```python
from build123d import *

# Parameters (mm, degrees)
SKETCH_1_W          = 320
SKETCH_1_H          = 121
EXTRUDE_1_DEPTH     = 4
SKETCH_2_W          = 5
SKETCH_2_H          = 30
CUT_EXTRUDE_1_DEPTH = 343.135937896
SKETCH_3_R          = 1.5
CUT_EXTRUDE_2_DEPTH = 343.135937896
SKETCH_4_R          = 1.5
CUT_EXTRUDE_3_DEPTH = 343.135937896
SKETCH_6_R          = 2
CUT_EXTRUDE_5_DEPTH = 343.135937896
SKETCH_5_W          = 250
SKETCH_5_H          = 30
CUT_EXTRUDE_4_DEPTH = 343.135937896


with BuildPart() as part:
    # 草图1 → 凸台-拉伸1 (new body)
    with BuildSketch(Plane.XY):
        with Locations((160, 60.5)):
            Rectangle(SKETCH_1_W, SKETCH_1_H)
    extrude(amount=EXTRUDE_1_DEPTH)

    # 草图2 → 切除-拉伸1 (cut, through all)
    with BuildSketch(Plane.XY.offset(4)):
        with Locations((32.5, 15)):
            Rectangle(SKETCH_2_W, SKETCH_2_H)
        with Locations((287.5, 15)):
            Rectangle(SKETCH_2_W, SKETCH_2_H)
    extrude(amount=-CUT_EXTRUDE_1_DEPTH, mode=Mode.SUBTRACT)

    # 草图3 → 切除-拉伸2 (cut, through all)
    with BuildSketch(Plane.XY.offset(4)):
        with Locations((40, 116)):
            Circle(SKETCH_3_R)
        with Locations((60, 116)):
            Circle(SKETCH_3_R)
        with Locations((140, 116)):
            Circle(SKETCH_3_R)
        with Locations((160, 116)):
            Circle(SKETCH_3_R)
        with Locations(Location((260, 116, 0), (0, 0, 180))):
            Circle(SKETCH_3_R)
        with Locations(Location((280, 116, 0), (0, 0, 180))):
            Circle(SKETCH_3_R)
        with Locations(Location((180, 116, 0), (0, 0, 180))):
            Circle(SKETCH_3_R)
    extrude(amount=-CUT_EXTRUDE_2_DEPTH, mode=Mode.SUBTRACT)

    # 草图4 → 切除-拉伸3 (cut, through all)
    with BuildSketch(Plane.XY.offset(4)):
        with Locations((5, 90)):
            Circle(SKETCH_4_R)
        with Locations((25, 90)):
            Circle(SKETCH_4_R)
        with Locations((5, 10)):
            Circle(SKETCH_4_R)
        with Locations((25, 10)):
            Circle(SKETCH_4_R)
        with Locations(Location((295, 10, 0), (0, 0, 180))):
            Circle(SKETCH_4_R)
        with Locations(Location((315, 10, 0), (0, 0, 180))):
            Circle(SKETCH_4_R)
        with Locations(Location((295, 90, 0), (0, 0, 180))):
            Circle(SKETCH_4_R)
        with Locations(Location((315, 90, 0), (0, 0, 180))):
            Circle(SKETCH_4_R)
    extrude(amount=-CUT_EXTRUDE_3_DEPTH, mode=Mode.SUBTRACT)

    # 草图6 → 切除-拉伸5 (cut, through all)
    with BuildSketch(Plane.XY.offset(4)):
        with Locations((112.5, 75.5)):
            Circle(SKETCH_6_R)
        with Locations((207.5, 75.5)):
            Circle(SKETCH_6_R)
        with Locations((207.5, 50.5)):
            Circle(SKETCH_6_R)
        with Locations((112.5, 50.5)):
            Circle(SKETCH_6_R)
        with BuildLine():
            Line((127.5, 70), (192.5, 70))
            ThreePointArc((192.5, 70), (199.5, 63), (192.5, 56))
            Line((192.5, 56), (127.5, 56))
            ThreePointArc((127.5, 56), (120.5, 63), (127.5, 70))
        make_face()
    extrude(amount=-CUT_EXTRUDE_5_DEPTH, mode=Mode.SUBTRACT)

    # 草图5 → 切除-拉伸4 (cut, through all)
    with BuildSketch(Plane.XY.offset(4)):
        with BuildLine():
            Line((5, 101.368043607), (5, 114.5))
            ThreePointArc((5, 114.5), (5.439339828, 115.560660172), (6.5, 116))
            Line((6.5, 116), (21.091062659, 116))
            ThreePointArc((21.091062659, 116), (22.491493276, 115.037395651), (22.094509756, 113.385058781))
            Line((22.094509756, 113.385058781), (7.503447097, 100.253102388))
            ThreePointArc((7.503447097, 100.253102388), (5.889742123, 99.997793512), (5, 101.368043607))
        make_face()
        with BuildLine():
            Line((22, 75), (22, 45))
            ThreePointArc((22, 45), (15, 38), (8, 45))
            Line((8, 45), (8, 75))
            ThreePointArc((8, 75), (15, 82), (22, 75))
        make_face()
        with BuildLine():
            Line((38.908937341, 85), (56.833333333, 85))
            ThreePointArc((56.833333333, 85), (57.893993505, 85.439339828), (58.333333333, 86.5))
            Line((58.333333333, 86.5), (58.333333333, 102.631956393))
            ThreePointArc((58.333333333, 102.631956393), (57.443591211, 104.002206488), (55.829886236, 103.746897612))
            Line((55.829886236, 103.746897612), (37.905490244, 87.614941219))
            ThreePointArc((37.905490244, 87.614941219), (37.508506724, 85.962604349), (38.908937341, 85))
        make_face()
        with BuildLine():
            Line((35, 68.5), (35, 47.25))
            ThreePointArc((35, 47.25), (35.667949706, 46.001924558), (37.076923077, 45.865384615))
            Line((37.076923077, 45.865384615), (88.076923077, 67.115384615))
            ThreePointArc((88.076923077, 67.115384615), (88.970871014, 68.794174203), (87.5, 70))
            Line((87.5, 70), (36.5, 70))
            ThreePointArc((36.5, 70), (35.439339828, 69.560660172), (35, 68.5))
        make_face()
        with Locations((160, 15)):
            Rectangle(SKETCH_5_W, SKETCH_5_H)
        with BuildLine():
            Line((81.5, 45), (101, 45))
            ThreePointArc((101, 45), (102.060660172, 45.439339828), (102.5, 46.5))
            Line((102.5, 46.5), (102.5, 54.625))
            ThreePointArc((102.5, 54.625), (101.832050294, 55.873075442), (100.423076923, 56.009615385))
            Line((100.423076923, 56.009615385), (80.923076923, 47.884615385))
            ThreePointArc((80.923076923, 47.884615385), (80.029128986, 46.205825797), (81.5, 45))
        make_face()
        with BuildLine():
            Line((68.333333333, 87.256929624), (68.333333333, 104.5))
            ThreePointArc((68.333333333, 104.5), (68.772673162, 105.560660172), (69.833333333, 106))
            Line((69.833333333, 106), (110.888262801, 106))
            ThreePointArc((110.888262801, 106), (112.358715068, 104.796260242), (111.469111528, 103.117026842))
            Line((111.469111528, 103.117026842), (70.41418206, 85.873956465))
            ThreePointArc((70.41418206, 85.873956465), (69.00305419, 86.007675228), (68.333333333, 87.256929624))
        make_face()
        with BuildLine():
            Line((111.788920254, 84.01540935), (153.193641955, 75.376872258))
            ThreePointArc((153.193641955, 75.376872258), (154.446166722, 75.68130869), (155, 76.845253935))
            Line((155, 76.845253935), (155, 102.873774141))
            ThreePointArc((155, 102.873774141), (154.330279143, 104.123028536), (152.919151273, 104.256747299))
            Line((152.919151273, 104.256747299), (111.514429572, 86.866764185))
            ThreePointArc((111.514429572, 86.866764185), (110.602180826, 85.340055375), (111.788920254, 84.01540935))
        make_face()
        with BuildLine():
            Line((167.080848727, 104.256747299), (208.485570428, 86.866764185))
            ThreePointArc((208.485570428, 86.866764185), (209.397819174, 85.340055375), (208.211079746, 84.01540935))
            Line((208.211079746, 84.01540935), (166.806358045, 75.376872258))
            ThreePointArc((166.806358045, 75.376872258), (165.553833278, 75.68130869), (165, 76.845253935))
            Line((165, 76.845253935), (165, 102.873774141))
            ThreePointArc((165, 102.873774141), (165.669720857, 104.123028536), (167.080848727, 104.256747299))
        make_face()
        with BuildLine():
            Line((208.530888472, 103.117026842), (249.58581794, 85.873956465))
            ThreePointArc((249.58581794, 85.873956465), (250.99694581, 86.007675228), (251.666666667, 87.256929624))
            Line((251.666666667, 87.256929624), (251.666666667, 104.5))
            ThreePointArc((251.666666667, 104.5), (251.227326838, 105.560660172), (250.166666667, 106))
            Line((250.166666667, 106), (209.111737199, 106))
            ThreePointArc((209.111737199, 106), (207.641284932, 104.796260242), (208.530888472, 103.117026842))
        make_face()
        with BuildLine():
            Line((219.576923077, 56.009615385), (239.076923077, 47.884615385))
            ThreePointArc((239.076923077, 47.884615385), (239.970871014, 46.205825797), (238.5, 45))
            Line((238.5, 45), (219, 45))
            ThreePointArc((219, 45), (217.939339828, 45.439339828), (217.5, 46.5))
            Line((217.5, 46.5), (217.5, 54.625))
            ThreePointArc((217.5, 54.625), (218.167949706, 55.873075442), (219.576923077, 56.009615385))
        make_face()
        with BuildLine():
            Line((232.5, 70), (283.5, 70))
            ThreePointArc((283.5, 70), (284.560660172, 69.560660172), (285, 68.5))
            Line((285, 68.5), (285, 47.25))
            ThreePointArc((285, 47.25), (284.332050294, 46.001924558), (282.923076923, 45.865384615))
            Line((282.923076923, 45.865384615), (231.923076923, 67.115384615))
            ThreePointArc((231.923076923, 67.115384615), (231.029128986, 68.794174203), (232.5, 70))
        make_face()
        with BuildLine():
            Line((264.170113764, 103.746897612), (282.094509756, 87.614941219))
            ThreePointArc((282.094509756, 87.614941219), (282.491493276, 85.962604349), (281.091062659, 85))
            Line((281.091062659, 85), (263.166666667, 85))
            ThreePointArc((263.166666667, 85), (262.106006495, 85.439339828), (261.666666667, 86.5))
            Line((261.666666667, 86.5), (261.666666667, 102.631956393))
            ThreePointArc((261.666666667, 102.631956393), (262.556408789, 104.002206488), (264.170113764, 103.746897612))
        make_face()
        with BuildLine():
            Line((297.905490244, 113.385058781), (312.496552903, 100.253102388))
            ThreePointArc((312.496552903, 100.253102388), (314.110257877, 99.997793512), (315, 101.368043607))
            Line((315, 101.368043607), (315, 114.5))
            ThreePointArc((315, 114.5), (314.560660172, 115.560660172), (313.5, 116))
            Line((313.5, 116), (298.908937341, 116))
            ThreePointArc((298.908937341, 116), (297.508506724, 115.037395651), (297.905490244, 113.385058781))
        make_face()
        with BuildLine():
            Line((298, 75), (298, 45))
            ThreePointArc((298, 45), (305, 38), (312, 45))
            Line((312, 45), (312, 75))
            ThreePointArc((312, 75), (305, 82), (298, 75))
        make_face()
        with BuildLine():
            Line((12.143074903, 15), (18.5, 15))
            ThreePointArc((18.5, 15), (19.560660172, 15.439339828), (20, 16.5))
            Line((20, 16.5), (20, 21.797437581))
            ThreePointArc((20, 21.797437581), (19.136233094, 23.155821713), (17.539723401, 22.9497695))
            Line((17.539723401, 22.9497695), (11.182798303, 17.652331919))
            ThreePointArc((11.182798303, 17.652331919), (10.732667536, 15.989362104), (12.143074903, 15))
        make_face()
        with BuildLine():
            Line((302.460276599, 22.9497695), (308.817201697, 17.652331919))
            ThreePointArc((308.817201697, 17.652331919), (309.267332464, 15.989362104), (307.856925097, 15))
            Line((307.856925097, 15), (301.5, 15))
            ThreePointArc((301.5, 15), (300.439339828, 15.439339828), (300, 16.5))
            Line((300, 16.5), (300, 21.797437581))
            ThreePointArc((300, 21.797437581), (300.863766906, 23.155821713), (302.460276599, 22.9497695))
        make_face()
    extrude(amount=-CUT_EXTRUDE_4_DEPTH, mode=Mode.SUBTRACT)


solid = part.part
```
Could you check a few things on this model? Use its own coordinates, in mm. Round coordinates to 2 decimals unless told otherwise and drop trailing zeros. Loops run counter-clockwise (first coordinate to the right, second up) from the corner with the lowest first, then second, coordinate; pieces in that order, holes last. Notation, with made-up numbers: M 83.25,-25 L 120.25,-25 A14 ccw 120.25,-12 Z; hole C 23.25,-11 d10. An arc over 180 degrees is marked long. Put each result on its own line as item: value.
Q1. Imagine slicing it at B-B (z = 2.6). State how many separate pieces and enclosed holes the cut face has, then the cut area to 3 significant figures.
Check result:
separate pieces: 1
enclosed holes: 36
area: 23,400 mm2
Q2. Imagine slicing it at A-A (y = 26.5). Write out the boundary of the cut face in (x, z), then the cut area to 3 significant figures.
Check result:
outline: M 0,0 L 30,0 L 30,4 L 0,4 Z; M 290,0 L 320,0 L 320,4 L 290,4 Z
area: 240 mm2
Q3. Imagine slicing it at C-C (x = 124.5). Write out the boundary of the cut face in (y, z), then the cut area to 3 significant figures.
Check result:
outline: M 30,0 L 56.68,0 L 56.68,4 L 30,4 Z; M 69.32,0 L 81.36,0 L 81.36,4 L 69.32,4 Z; M 92.32,0 L 121,0 L 121,4 L 92.32,4 Z
area: 270 mm2
Q4. I need wall thicknesses on probe 1 along Y at (x, z) = (25, 2.4); probe 2 along X at (y, z) = (19, 2.65); probe 3 along Y at (x, z) = (112.5, 2.25). Which ranges of each line are inside material? Lowest first, please.
Check result:
probe 1: 0 to 8.5, 11.5 to 88.5, 91.5 to 121
probe 2: 0 to 12.8, 20 to 30, 290 to 300, 307.2 to 320
probe 3: 30 to 48.5, 52.5 to 73.5, 77.5 to 83.87, 87.28 to 121
